Build history of the part. All positions in model axes, mm. A direction names the side the tool comes from. Give positions to 0.01 mm unless a question says otherwise; leave off trailing zeros. Loops run counter-clockwise (first coordinate to the right, second up) from the corner with the lowest first, then second, coordinate; pieces in that order, holes last. Notation, with made-up numbers: (5, -40) -> (45, -40) arc R18 cw to (45, -19) -> close; hole circle Ø1 at (54, -19). An arc over 180 degrees is marked (long way). Answer as a JSON object with one key per item and string values. Group by question number.
Q1. Drop flat-ended pins along their axis: pin 1 (6 mm diameter, centred on x = 14, z = 43, fed in from -Y); pin 2 (12 mm diameter, centred on y = -13, z = 42.5, fed in from +X); pin 3 (3 mm diameter, centred on x = -23, y = -21, fed in from +Z). Give the stop position or say it passes through.
Q2. Tool access for faces 4 (the flat face through (-25.39, -14.648, 3.296)), 5 (the cylindrical face through (-22.681, -33.264, 4.573)), 6 (the cylindrical face through (11.974, -28.353, 18.369)): list every direction of +Z, -Z, +X, -X, +Y, -Y with a clear straight run to the whole face (end or side of a thin tool).
Q3. Wall check: probe 1 along Z at (x, y) = (9.99, -27.5); probe 2 along Z at (x, y) = (-33.5, -15); probe 3 along X at (y, z) = (-20, 26). Give the ranges that are in metal, low to high. Write a range as from..to.
Q4. Two-plate mould, pull along X, no slides. Class faces 1 (the conical face through (9.93, -20.85, 20.32)), 2 (the flat face through (0, 0, 9)), 3 (the flat face through (-28.863, -14.648, 26.096)): pulls with the +X half, pulls with the -X half, needs draft (parallel to the pull), parting line crosses it, or undercut.
Q5. Band-saw the part on A-A, the plane y = -9.5. Write the cut outline in (x, z).
from build123d import *

# Parameters (mm, degrees)
F1_DEPTH = 34.79205
F2_R     = 5.08
F4_D     = 5
F4_DEPTH = 12.7
F4_TIP   = 1.5021515476


with BuildPart() as f1:
    # F0 (on Front) → F1 (new body)
    with BuildSketch(Plane.XZ):
        Polygon((8.8970496238, 50.7587020687), (-43.8900001305, 32.1299992502), (-13.4100001305, 19.8900010437), (-37.7099998295, -13.7700010091), (44.3699993193, -19.1700011492), align=None)
    extrude(amount=F1_DEPTH)

    # F2
    f2_edges = [f1.edges().sort_by_distance(p)[0] for p in [
        (-17.496475, -34.79205, 41.444351),
        (26.633524, -34.79205, 15.79435),
        (3.33, -34.79205, -16.470001),
        (-25.56, -34.79205, 3.06),
        (-28.65, -34.79205, 26.01),
    ]]
    fillet(f2_edges, radius=F2_R)

    # F4
    with Locations(Plane.XZ.offset(34.79205)):
        with Locations((9.9899992347, 19.8900010437)):
            Hole(F4_D / 2, depth=F4_DEPTH)
            with Locations((0, 0, -(F4_DEPTH + F4_TIP / 2))):  # 118° drill point
                Cone(0, F4_D / 2, F4_TIP, mode=Mode.SUBTRACT)


solid = f1.part
Worked answers:
{
 "1": {"pin 1": "y = -33.72", "pin 2": "x = 16.13", "pin 3": "z = 40.03"},
 "2": {"face 4": "-X, +Y, -Y", "face 5": "-X, -Y", "face 6": "-Y"},
 "3": {"probe 1": "-16.91..17.39, 22.39..48.6", "probe 2": "-14.05..-7.94, 27.96..35.8", "probe 3": "-28.63..21.46"},
 "4": {"face 1": "undercut", "face 2": "needs draft", "face 3": "pulls with the -X half"},
 "5": {"outline": "(-43.89, 32.13) -> (-13.41, 19.89) -> (-37.71, -13.77) -> (44.37, -19.17) -> (8.9, 50.76) -> close"}
}
